```python
from build123d import *

# Parameters (mm, degrees)
BOSS_EXTRUDE1_DEPTH = 30
SKETCH2_R           = 7
SKETCH2_R_2         = 1.5
CUT_EXTRUDE1_DEPTH  = 55
SKETCH3_R           = 3
CUT_EXTRUDE2_DEPTH  = 55
SKETCH4_W           = 8
SKETCH4_H           = 40
BOSS_EXTRUDE2_DEPTH = 60
SKETCH5_R           = 2.5
CUT_EXTRUDE3_DEPTH  = 10


with BuildPart() as part:
    # Sketch1 → Boss-Extrude1 (new, symmetric)
    with BuildSketch(Plane(origin=(0, 0, 0), x_dir=(0, 0, -1), z_dir=(1, 0, 0))):
        Polygon((0, 50), (0, 0), (-52, 0), (-52, -8), (8, -8), (8, 50), align=None)
    extrude(amount=BOSS_EXTRUDE1_DEPTH, both=True)

    # Sketch2 → Cut-Extrude1 (cut)
    with BuildSketch(Plane(origin=(0, 0, 0), x_dir=(1, 0, 0), z_dir=(0, 1, 0))):
        with Locations(Location((0, -37, 0), (0, 0, 270))):
            Circle(SKETCH2_R)
        with Locations(Location((15.75, -30, 0), (0, 0, 270))):
            Circle(SKETCH2_R_2)
        with Locations(Location((7.875, -43.63990011, 0), (0, 0, 270))):
            Circle(SKETCH2_R_2)
        with Locations(Location((-7.875, -43.63990011, 0), (0, 0, 270))):
            Circle(SKETCH2_R_2)
        with Locations(Location((-15.75, -30, 0), (0, 0, 270))):
            Circle(SKETCH2_R_2)
        with Locations(Location((-7.875, -16.36009989, 0), (0, 0, 270))):
            Circle(SKETCH2_R_2)
        with Locations(Location((7.875, -16.36009989, 0), (0, 0, 270))):
            Circle(SKETCH2_R_2)
    extrude(amount=-CUT_EXTRUDE1_DEPTH, mode=Mode.SUBTRACT)

    # Sketch3 → Cut-Extrude2 (cut)
    with BuildSketch(Plane.XY):
        with Locations((0, 45)):
            Circle(SKETCH3_R)
    extrude(amount=-CUT_EXTRUDE2_DEPTH, mode=Mode.SUBTRACT)

    # Sketch4 → Boss-Extrude2 (add)
    with BuildSketch(Plane(origin=(30, 0, 0), x_dir=(0, 0, -1), z_dir=(1, 0, 0))):
        with Locations((-56, -20)):
            Rectangle(SKETCH4_W, SKETCH4_H)
    extrude(amount=-BOSS_EXTRUDE2_DEPTH)

    # Sketch5 → Cut-Extrude3 (cut)
    with BuildSketch(Plane.XY.offset(60)):
        with Locations((25, -33.45)):
            Circle(SKETCH5_R)
        with Locations((-25, -33.45)):
            Circle(SKETCH5_R)
    extrude(amount=-CUT_EXTRUDE3_DEPTH, mode=Mode.SUBTRACT)


solid = part.part
```
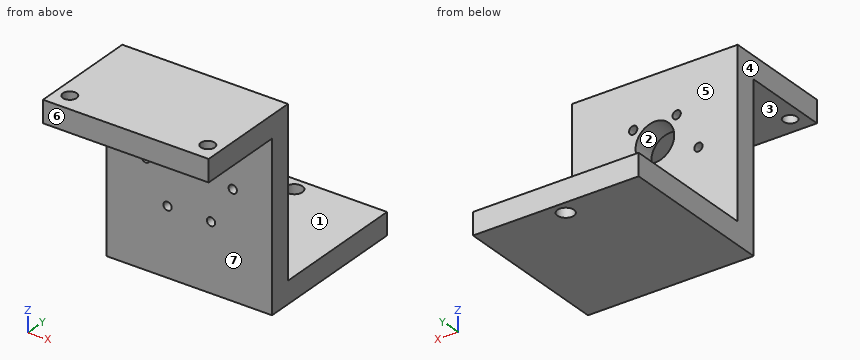
Here's how the part is built. I have some questions about the finished solid (model axes, mm). Face numbers are marked on the shaded views. A direction names the side the tool comes from. Give positions to 0.01 mm unless a question says otherwise; leave off trailing zeros. Write each loop counter-clockwise with the first axis right and the second up, starting at its lowest first coordinate (ties: lowest second). Pieces come first, ordered by that corner, then holes. Notation, with made-up numbers: M -23,43 L 27,43 A13 ccw 27,54 Z; hole C -24,56.5 d3. An arc over 180 degrees is marked long. Put each result on its own line as item: value. Start each with the question number.
Item 1: If we section it at D-D, the plane x = -25: Write out the boundary of the cut face in (y, z).
Item 2: If we section it at B-B, the plane z = 37: Write out the boundary of the cut face in (x, y), then the cut area to 3 significant figures.
Item 3: Will these pins go through, and if not, where does the flat tip stop? pin 1 (16 mm diameter, centred on x = -9.5, y = -17.5, fed in from -Z); pin 2 (1 mm diameter, centred on x = 0.5, z = 9.5, fed in from +Y); pin 3 (10 mm diameter, centred on x = 2.5, z = 18, fed in from -Y); pin 4 (7 mm diameter, centred on x = 0, y = 45, fed in from -Z).
Item 4: Thinking about a two-plate mould opening in Z: for the marked faces 1, 2, 3 and 4, which applies, +Z half, -Z half, draft (parallel to the pull), parting line (faces both ways), or undercut?
Item 5: If we section it at C-C, the plane x = 0: Write out the boundary of the cut face in (y, z), then the cut area to 3 significant figures.
Item 6: On a 3-axis mill with a long thin cutter (end or side, diameter ignored), from which of +Z, -Z, +X, -X, +Y, -Y can I reach the whole of each face in a straight line? I mean the marked faces 5, 6 and 7. Say none if no direction works.
Item 7: If we section it at A-A, the plane y = -33.45: Write out the boundary of the cut face in (x, z).
Item 8: I need wall thicknesses on L1, parallel to Y at x = 25, z = 57; L2, parallel to Z at x = 9, y = -33; L3, parallel to Z at x = 9, y = 36. Which ranges of each line are inside material? Lowest first, please. Write a range as from..to.
Values:
1. outline: M -40,52 L -35.95,52 L -35.95,60 L -40,60 Z; M -30.95,52 L -8,52 L -8,-8 L 50,-8 L 50,0 L 0,0 L 0,60 L -30.95,60 Z
2. outline: M -30,-8 L -7,-8 L -7,0 L -30,0 Z; M 7,-8 L 30,-8 L 30,0 L 7,0 Z
2. area: 368 mm²
3. pin 1: z = 52
3. pin 2: y = 0
3. pin 3: y = -8
3. pin 4: z = -8
4. face 1: +Z half
4. face 2: undercut
4. face 3: -Z half
4. face 4: draft
5. outline: M -40,52 L -8,52 L -8,44 L 0,44 L 0,60 L -40,60 Z; M -8,-8 L 42,-8 L 42,0 L 0,0 L 0,30 L -8,30 Z; M 48,-8 L 50,-8 L 50,0 L 48,0 Z
5. area: 1,040 mm²
6. face 5: +Z, +X, -X, +Y
6. face 6: +Z, -Z, +X, -X, -Y
6. face 7: -Z, +X, -X, -Y
7. outline: M -30,52 L -27.5,52 L -27.5,60 L -30,60 Z; M -22.5,52 L 22.5,52 L 22.5,60 L -22.5,60 Z; M 27.5,52 L 30,52 L 30,60 L 27.5,60 Z
8. L1: -40..-35.95, -30.95..0
8. L2: 52..60
8. L3: -8..0
